Geometry: see drawing. Coordinates: mm, zero at the bounding-box minimum. A direction names the side the tool comes from. Coordinates: 2 decimals unless noted, no trailing zeros. Write each loop counter-clockwise with the first axis right and the second up, starting at its lowest first coordinate (ties: lowest second). Pieces come first, ordered by that corner, then holes. Notation, with made-up numbers: (33.25, 83.25) - (77.25, 83.25) arc R15 ccw to (77.25, 101.25) - close; hole circle Ø11 at (33.5, -18). An arc over 180 degrees is marked (long way). Use a Markdown table: item, result. Add a question column.
Q1. Section query D-D (z = 48). Return the cut outline in (x, y).
Q2. Section query B-B (y = 19.5). Return the cut outline in (x, z), then the cut area to 3 significant figures.
Q3. Section query C-C (x = 30). Return the cut outline in (y, z), then the cut area to 3 significant figures.
Q4. Pin query (flat end, axial travel): P1, Ø1.5, axis at y = 20, z = 21.5, coming from the +X side; P2, Ø11, axis at x = 16.5, y = 14.5, coming from the -Z side; P3, Ø16, axis at x = 32.5, z = 35, coming from the +Y side. Return the tip coordinate at first contact, or that it passes through.
Q5. Material intervals for probe 1 along X at (y, z) = (3.5, 46); probe 2 along Z at (x, y) = (57, 21); probe 3 along Y at (x, z) = (33.5, 4.5), sorted ascending. Write a range as from..to.
Q6. Section query A-A (z = 24). Return the cut outline in (x, y), then the cut area to 3 significant figures.
Q7. Set-up query: the marked faces 1 and 2. Return all of +Z, -Z, +X, -X, +Y, -Y with unobstructed straight access to the full face (end or side cutting, diameter ignored); none if empty.
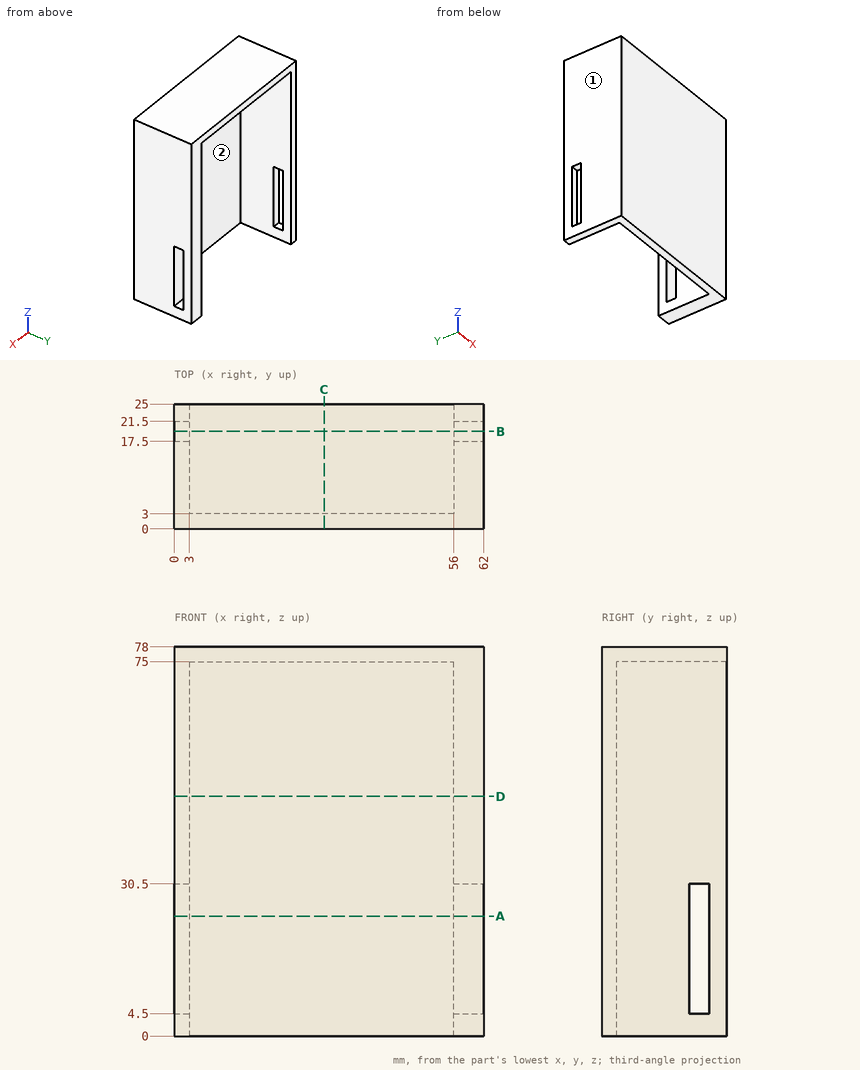
Values follow:
| question | item | result |
|---|---|---|
| 1 | outline | (0, 0) - (62, 0) - (62, 25) - (56, 25) - (56, 3) - (3, 3) - (3, 25) - (0, 25) - close |
| 2 | outline | (0, 0) - (3, 0) - (3, 4.5) - (0, 4.5) - close; (0, 30.5) - (3, 30.5) - (3, 75) - (56, 75) - (56, 30.5) - (62, 30.5) - (62, 78) - (0, 78) - close; (56, 0) - (62, 0) - (62, 4.5) - (56, 4.5) - close |
| 2 | area | 627 mm2 |
| 3 | outline | (0, 0) - (3, 0) - (3, 75) - (25, 75) - (25, 78) - (0, 78) - close |
| 3 | area | 300 mm2 |
| 4 | P1 | through |
| 4 | P2 | z = 75 |
| 4 | P3 | y = 3 |
| 5 | probe 1 | 0..3, 56..62 |
| 5 | probe 2 | 0..4.5, 30.5..78 |
| 5 | probe 3 | 0..3 |
| 6 | outline | (0, 0) - (62, 0) - (62, 17.5) - (56, 17.5) - (56, 3) - (3, 3) - (3, 17.5) - (0, 17.5) - close; (0, 21.5) - (3, 21.5) - (3, 25) - (0, 25) - close; (56, 21.5) - (62, 21.5) - (62, 25) - (56, 25) - close |
| 6 | area | 348 mm2 |
| 7 | face 1 | +Z, -Z, -X, +Y, -Y |
| 7 | face 2 | -Z, +Y |
